Can you work these out from the model? Positions are in its coordinate system, mm. Coordinates: 2 decimals unless noted, no trailing zeros. Order: outer loops, then holes, each group sorted by start corner. A loop starts at its lowest first (then second) coordinate and runs counter-clockwise, first axis right, second up. Notation, with made-up numbers: (28, 48) - (42, 48) arc R27 cw to (42, 77) - close; hole circle Ø3 at (77, 75.5). An arc over 180 degrees is marked (long way). Return JSON: item names as keys, results as strings. Group by question number.
1) Imagine slicing it at D-D (z = 1.55). Write out the boundary of the cut face in (x, y).
2) Imagine slicing it at A-A (y = -31). Write out the boundary of the cut face in (x, z), and give its area (3 significant figures).
3) Imagine slicing it at C-C (y = 0). Write out the boundary of the cut face in (x, z), and give its area (3 significant figures).
4) Imagine slicing it at B-B (x = 0). Write out the boundary of the cut face in (y, z).
5) If I drill on line 1 along Y through (x, z) = (15.5, 2.25); line 2 along X through (y, z) = (15, 1.7); line 3 along X through (y, z) = (-33, 1.1), over which ranges is the centre line in solid material (lowest first)?
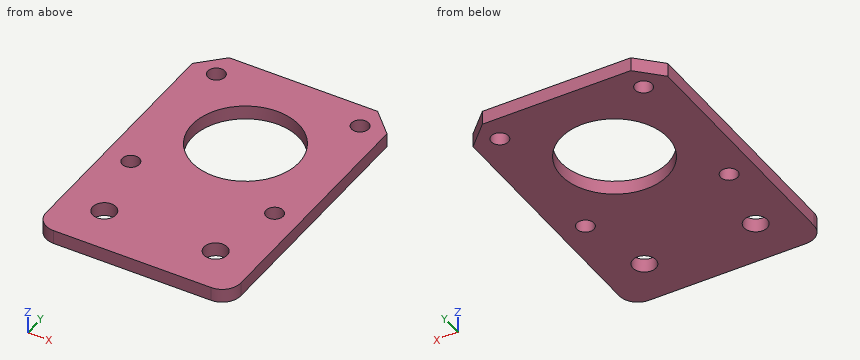
```python
from build123d import *

# Parameters (mm, degrees)
SKETCH_1_R      = 1.849740933
SKETCH_1_R_2    = 2.5
SKETCH_1_R_3    = 11.5
EXTRUDE_1_DEPTH = 3
FILLET_1_R      = 4
CHAMFER_1_SIZE  = 5


with BuildPart() as part:
    # 草圖1 → 填料-伸長1 (new body)
    with BuildSketch(Plane.XY):
        Polygon((-21, 21), (21, 21), (21, -21), (21, -41), (-21, -41), (-21, -21), align=None)
        with Locations((-15.5, 15.5)):
            Circle(SKETCH_1_R, mode=Mode.SUBTRACT)
        with Locations(Location((15.5, 15.5, 0), (0, 0, 180))):
            Circle(SKETCH_1_R, mode=Mode.SUBTRACT)
        with Locations((15.5, -15.5)):
            Circle(SKETCH_1_R, mode=Mode.SUBTRACT)
        with Locations(Location((-15.5, -15.5, 0), (0, 0, 180))):
            Circle(SKETCH_1_R, mode=Mode.SUBTRACT)
        with Locations((-12, -31)):
            Circle(SKETCH_1_R_2, mode=Mode.SUBTRACT)
        with Locations(Location((12, -31, 0), (0, 0, 180))):
            Circle(SKETCH_1_R_2, mode=Mode.SUBTRACT)
        Circle(SKETCH_1_R_3, mode=Mode.SUBTRACT)
    extrude(amount=EXTRUDE_1_DEPTH)

    # 圓角1
    fillet_1_edges = [part.edges().sort_by_distance(p)[0] for p in [
        (21, -41, 1.5),
        (-21, -41, 1.5),
    ]]
    fillet(fillet_1_edges, radius=FILLET_1_R)

    # 導角1
    chamfer_1_edges = [part.edges().sort_by_distance(p)[0] for p in [
        (-21, 21, 1.5),
        (21, 21, 1.5),
    ]]
    chamfer(chamfer_1_edges, length=CHAMFER_1_SIZE)


solid = part.part
```
Calculated:
{
 "1": {"outline": "(-21, -37) arc R4 ccw to (-17, -41) - (17, -41) arc R4 ccw to (21, -37) - (21, 16) - (16, 21) - (-16, 21) - (-21, 16) - close; hole circle Ø3.7 at (-15.5, -15.5); hole circle Ø3.7 at (-15.5, 15.5); hole circle Ø5 at (-12, -31); hole circle Ø23 at (0, 0); hole circle Ø5 at (12, -31); hole circle Ø3.7 at (15.5, -15.5); hole circle Ø3.7 at (15.5, 15.5)"},
 "2": {"outline": "(-21, 0) - (-14.5, 0) - (-14.5, 3) - (-21, 3) - close; (-9.5, 0) - (9.5, 0) - (9.5, 3) - (-9.5, 3) - close; (14.5, 0) - (21, 0) - (21, 3) - (14.5, 3) - close", "area": "96.0 mm2"},
 "3": {"outline": "(-21, 0) - (-11.5, 0) - (-11.5, 3) - (-21, 3) - close; (11.5, 0) - (21, 0) - (21, 3) - (11.5, 3) - close", "area": "57.0 mm2"},
 "4": {"outline": "(-41, 0) - (-11.5, 0) - (-11.5, 3) - (-41, 3) - close; (11.5, 0) - (21, 0) - (21, 3) - (11.5, 3) - close"},
 "5": {"line 1": "-41 to -17.35, -13.65 to 13.65, 17.35 to 21", "line 2": "-21 to -17.28, -13.72 to 13.72, 17.28 to 21", "line 3": "-21 to -13.5, -10.5 to 10.5, 13.5 to 21"}
}
